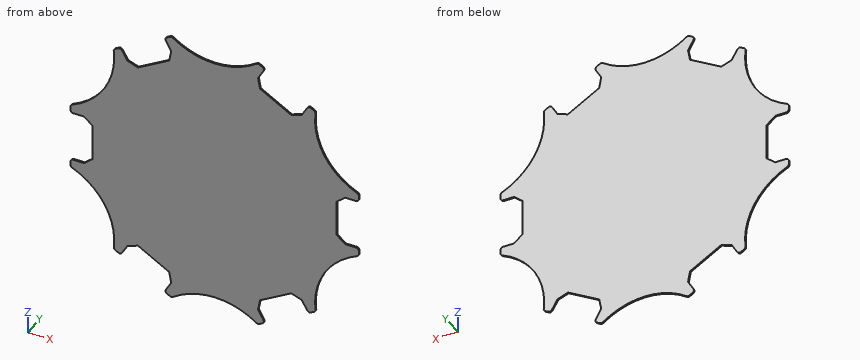
```python
from build123d import *

# Parameters (mm, degrees)
SKETCH2_R           = 1.35
BOSS_EXTRUDE1_DEPTH = 1
CIRPATTERN1_COUNT   = 6
CUT_EXTRUDE3_DEPTH  = 5
CUT_EXTRUDE9_DEPTH  = 10
CUT_EXTRUDE10_DEPTH = 186.676097905
FILLET2_R           = 2


with BuildPart() as part:
    # Sketch2 → Boss-Extrude1 (new body)
    with BuildSketch(Plane(origin=(0, 0, 0), x_dir=(1, 0, 0), z_dir=(0, 1, 0))):
        Polygon((0, 125), (-58.08143708, 125), (-35.58143708, 86.02885683), (-56.712456933, 73.82885683), (-79.212456933, 112.8), (-108.253175473, 62.5), (0, 0), align=None)
        with Locations(Location((-37.385731074, 81.753985699, 0), (0, 0, 270))):
            Circle(SKETCH2_R, mode=Mode.SUBTRACT)
        with Locations(Location((-52.108162939, 73.253985699, 0), (0, 0, 270))):
            Circle(SKETCH2_R, mode=Mode.SUBTRACT)
        with Locations(Location((-60.887328063, 75.459945743, 0), (0, 0, 270))):
            Circle(SKETCH2_R, mode=Mode.SUBTRACT)
        with Locations(Location((-34.90656595, 90.459945743, 0), (0, 0, 270))):
            Circle(SKETCH2_R, mode=Mode.SUBTRACT)
        with Locations(Location((-51.90656595, 119.904809472, 0), (0, 0, 270))):
            Circle(SKETCH2_R, mode=Mode.SUBTRACT)
        with Locations(Location((-43.40656595, 105.182377607, 0), (0, 0, 270))):
            Circle(SKETCH2_R, mode=Mode.SUBTRACT)
        with Locations(Location((-69.387328063, 90.182377607, 0), (0, 0, 270))):
            Circle(SKETCH2_R, mode=Mode.SUBTRACT)
        with Locations(Location((-77.887328063, 104.904809472, 0), (0, 0, 270))):
            Circle(SKETCH2_R, mode=Mode.SUBTRACT)
    boss_extrude1 = extrude(amount=BOSS_EXTRUDE1_DEPTH)

    # CirPattern1: Boss-Extrude1 ×6 about axis
    cirpattern1_axis = Axis((0, 0, 0), (0, 1, 0))
    for i in range(1, CIRPATTERN1_COUNT):
        add(boss_extrude1.rotate(cirpattern1_axis, i * 360 / CIRPATTERN1_COUNT))

    # Sketch4 → Cut-Extrude3 (cut)
    with BuildSketch(Plane(origin=(0, 1, 0), x_dir=(1, 0, 0), z_dir=(0, 1, 0))):
        with BuildLine():
            Line((79.212456933, -112.8), (137.293894013, -12.2))
            ThreePointArc((137.293894013, -12.2), (125.5592118, -23.716902798), (109.56410095, -27.524558982))
            ThreePointArc((109.56410095, -27.524558982), (77.942286341, -45), (78.619017782, -81.123015275))
            ThreePointArc((78.619017782, -81.123015275), (83.319046223, -96.879015699), (79.212456933, -112.8))
        make_face()
        with BuildLine():
            Line((137.293894013, 12.2), (79.212456933, 112.8))
            ThreePointArc((79.212456933, 112.8), (83.319046223, 96.879015699), (78.619017782, 81.123015275))
            ThreePointArc((78.619017782, 81.123015275), (77.942286341, 45), (109.56410095, 27.524558982))
            ThreePointArc((109.56410095, 27.524558982), (125.5592118, 23.716902798), (137.293894013, 12.2))
        make_face()
        with BuildLine():
            Line((58.08143708, 125), (-58.08143708, 125))
            ThreePointArc((-58.08143708, 125), (-42.240165578, 120.595918497), (-30.945083169, 108.647574257))
            ThreePointArc((-30.945083169, 108.647574257), (0, 90), (30.945083169, 108.647574257))
            ThreePointArc((30.945083169, 108.647574257), (42.240165578, 120.595918497), (58.08143708, 125))
        make_face()
        with BuildLine():
            Line((-79.212456933, 112.8), (-137.293894013, 12.2))
            ThreePointArc((-137.293894013, 12.2), (-125.5592118, 23.716902798), (-109.56410095, 27.524558982))
            ThreePointArc((-109.56410095, 27.524558982), (-77.942286341, 45), (-78.619017782, 81.123015275))
            ThreePointArc((-78.619017782, 81.123015275), (-83.319046223, 96.879015699), (-79.212456933, 112.8))
        make_face()
        with BuildLine():
            Line((-137.293894013, -12.2), (-79.212456933, -112.8))
            ThreePointArc((-79.212456933, -112.8), (-83.319046223, -96.879015699), (-78.619017782, -81.123015275))
            ThreePointArc((-78.619017782, -81.123015275), (-77.942286341, -45), (-109.56410095, -27.524558982))
            ThreePointArc((-109.56410095, -27.524558982), (-125.5592118, -23.716902798), (-137.293894013, -12.2))
        make_face()
        with BuildLine():
            Line((-58.08143708, -125), (58.08143708, -125))
            ThreePointArc((58.08143708, -125), (42.240165578, -120.595918497), (30.945083169, -108.647574257))
            ThreePointArc((30.945083169, -108.647574257), (0, -90), (-30.945083169, -108.647574257))
            ThreePointArc((-30.945083169, -108.647574257), (-42.240165578, -120.595918497), (-58.08143708, -125))
        make_face()
    extrude(amount=-CUT_EXTRUDE3_DEPTH, mode=Mode.SUBTRACT)

    # Sketch8 → Cut-Extrude9 (cut)
    with BuildSketch(Plane(origin=(0, 1, 0), x_dir=(1, 0, 0), z_dir=(0, 1, 0))):
        with BuildLine():
            Line((-79.627397697, 112.081427342), (-137.090413308, 12.563994028))
            ThreePointArc((-137.090413308, 12.563994028), (-131.312677504, 18.215244412), (-123.44128918, 20.048304088))
            ThreePointArc((-123.44128918, 20.048304088), (-77.942300503, 45.000018775), (-79.083064161, 96.879154221))
            ThreePointArc((-79.083064161, 96.879154221), (-81.425302856, 104.406169658), (-79.627397697, 112.081427342))
        make_face()
        with BuildLine():
            Line((-136.879097611, -12.918653567), (-79.425980046, -112.441801521))
            ThreePointArc((-79.425980046, -112.441801521), (-81.43123854, -104.612510346), (-79.083020624, -96.879158257))
            ThreePointArc((-79.083020624, -96.879158257), (-77.942345072, -45.000020873), (-123.441376125, -20.048383457))
            ThreePointArc((-123.441376125, -20.048383457), (-131.131082054, -18.31331395), (-136.879097611, -12.918653567))
        make_face()
        with BuildLine():
            Line((-57.251702025, -125.000120556), (57.66443115, -125.005835196))
            ThreePointArc((57.66443115, -125.005835196), (49.881436852, -122.827794405), (44.358266444, -116.927501992))
            ThreePointArc((44.358266444, -116.927501992), (-4.6681e-05, -90.000079294), (-44.358314075, -116.927577326))
            ThreePointArc((-44.358314075, -116.927577326), (-49.70578131, -122.719523255), (-57.251702025, -125.000120556))
        make_face()
        with BuildLine():
            Line((79.627393474, -112.081506636), (137.090409084, -12.564073322))
            ThreePointArc((137.090409084, -12.564073322), (131.312673281, -18.215323706), (123.441284957, -20.048383382))
            ThreePointArc((123.441284957, -20.048383382), (77.94229628, -45.000098069), (79.083059938, -96.879233516))
            ThreePointArc((79.083059938, -96.879233516), (81.425298632, -104.406248952), (79.627393474, -112.081506636))
        make_face()
        with BuildLine():
            Line((136.879093387, 12.918574273), (79.425975823, 112.441722226))
            ThreePointArc((79.425975823, 112.441722226), (81.431234317, 104.612431052), (79.083016401, 96.879078963))
            ThreePointArc((79.083016401, 96.879078963), (77.942340849, 44.999941578), (123.441371902, 20.048304163))
            ThreePointArc((123.441371902, 20.048304163), (131.131077831, 18.313234656), (136.879093387, 12.918574273))
        make_face()
        with BuildLine():
            Line((57.251697801, 125.000041262), (-57.664435373, 125.005755901))
            ThreePointArc((-57.664435373, 125.005755901), (-49.881441076, 122.827715111), (-44.358270668, 116.927422698))
            ThreePointArc((-44.358270668, 116.927422698), (4.2458e-05, 90), (44.358309852, 116.927498031))
            ThreePointArc((44.358309852, 116.927498031), (49.705777087, 122.71944396), (57.251697801, 125.000041262))
        make_face()
    extrude(amount=-CUT_EXTRUDE9_DEPTH, mode=Mode.SUBTRACT)

    # Sketch9 → Cut-Extrude10 (cut, through all)
    with BuildSketch(Plane(origin=(0, 1, 0), x_dir=(1, 0, 0), z_dir=(0, 1, 0))):
        Polygon((86.593894013, 12.8), (92.594856816, 17.9), (102.293894013, 17.9), (102.293894013, 27.495537581), (142.49088479, 27.495537581), (142.49088479, -27.407665194), (102.293894013, -27.407665194), (102.293894013, -17.9), (92.594856816, -17.9), (86.593894013, -12.8), align=None)
        Polygon((95.057276431, -109.652957246), (47.509708079, -137.104558633), (27.41121269, -102.292943464), (35.645092279, -97.539110868), (30.79557368, -89.139498262), (32.211821838, -81.392512028), (54.382072175, -68.592512028), (61.799283136, -71.239498262), (66.648801734, -79.639110868), (74.958781042, -74.841342077), align=None)
        Polygon((-47.43360836, -137.148494826), (-94.981176711, -109.696893439), (-74.882681323, -74.885278271), (-66.648801734, -79.639110868), (-61.799283136, -71.239498262), (-54.382072175, -68.592512028), (-32.211821838, -81.392512028), (-30.79557368, -89.139498262), (-35.645092279, -97.539110868), (-27.335112971, -102.336879658), align=None)
        Polygon((-142.49088479, -27.495537581), (-142.49088479, 27.407665194), (-102.293894013, 27.407665194), (-102.293894013, 17.9), (-92.594856816, 17.9), (-86.593894013, 12.8), (-86.593894013, -12.8), (-92.594856816, -17.9), (-102.293894013, -17.9), (-102.293894013, -27.495537581), align=None)
        Polygon((-95.057276431, 109.652957246), (-47.509708079, 137.104558633), (-27.41121269, 102.292943464), (-35.645092279, 97.539110868), (-30.79557368, 89.139498262), (-32.211821838, 81.392512028), (-54.382072175, 68.592512028), (-61.799283136, 71.239498262), (-66.648801734, 79.639110868), (-74.958781042, 74.841342077), align=None)
        Polygon((47.43360836, 137.148494826), (94.981176711, 109.696893439), (74.882681323, 74.885278271), (66.648801734, 79.639110868), (61.799283136, 71.239498262), (54.382072175, 68.592512028), (32.211821838, 81.392512028), (30.79557368, 89.139498262), (35.645092279, 97.539110868), (27.335112971, 102.336879658), align=None)
    extrude(amount=-CUT_EXTRUDE10_DEPTH, mode=Mode.SUBTRACT)

    # Fillet2
    fillet2_edges = [part.edges().sort_by_distance(p)[0] for p in [
        (30.596139754, 0.5, -100.454124967),
        (-30.596139754, 0.5, -100.454124967),
        (71.697787846, 0.5, -76.724077377),
        (102.293894013, 0.5, -23.730020176),
        (102.293894013, 0.5, 23.730102263),
        (71.697775448, 0.5, 76.724084535),
        (30.596078644, 0.5, 100.454160249),
        (-30.596083481, 0.5, 100.454157456),
        (-71.697781783, 0.5, 76.724080878),
        (-102.293894013, 0.5, 23.7301012),
        (-71.697789343, 0.5, -76.724076512),
        (-102.293894013, 0.5, -23.730024698),
        (66.648801734, 0.5, 79.639110868),
        (35.645092279, 0.5, 97.539110868),
        (-35.645092279, 0.5, 97.539110868),
        (-66.648801734, 0.5, 79.639110868),
        (-102.293894013, 0.5, 17.9),
        (-102.293894013, 0.5, -17.9),
        (-66.648801734, 0.5, -79.639110868),
        (-35.645092279, 0.5, -97.539110868),
        (35.645092279, 0.5, -97.539110868),
        (66.648801734, 0.5, -79.639110868),
        (102.293894013, 0.5, -17.9),
        (102.293894013, 0.5, 17.9),
    ]]
    fillet(fillet2_edges, radius=FILLET2_R)


solid = part.part
```
Check sheet for the modelled part. Datum: model origin and axes. Units: mm. Give positions to 0.01 mm unless a question says otherwise; leave off trailing zeros. Loops run counter-clockwise (first coordinate to the right, second up) from the corner with the lowest first, then second, coordinate; pieces in that order, holes last. Notation, with made-up numbers: M -8.5,80 L 27.5,80 A26 cw 27.5,117 Z; hole C 69.5,-35.5 d4. An arc over 180 degrees is marked long. Answer in a Markdown table with one row per item.
1) Thickness scan on line 1 (X direction, y = 0.7, z = -78); line 2 (X direction, y = 0.9, z = 2); line 3 (Z direction, x = 90, y = 0.4). Record the ranges inside material, lowest first.
Solutions:
| item | result |
|---|---|
| line 1 | x = -69.49 to -65.71, -38.09 to 38.09, 65.71 to 69.49 |
| line 2 | x = -86.59 to 86.59 |
| line 3 | z = -30.96 to -15.69, 15.69 to 30.96 |
2) Cross-section at B-B (x = -12). Enter the section's corners in (y, z).
Solutions:
| item | result |
|---|---|
| outline | M 0,-91.46 L 1,-91.46 L 1,91.46 L 0,91.46 Z |
3) Depth check by flat-ended pin: pin 1 (6 mm diameter, centred on x = -69, z = -40.5, fed in from -Y); pin 2 (0.5 mm diameter, centred on x = 95.5, y = 0.5, fed in from +Z). Enter the tip coordinate at first touch or a pass-through.
Solutions:
| item | result |
|---|---|
| pin 1 | stops at y = 0 |
| pin 2 | stops at z = 27.29 |
4) Cross-section at A-A (z = -2). Enter the section's corners in (x, y), plus the area to 3 significant figures.
Solutions:
| item | result |
|---|---|
| outline | M -86.59,0 L 86.59,0 L 86.59,1 L -86.59,1 Z |
| area | 173 mm^2 |
